Work out the finished part from the listing and answer in its coordinate system (mm). Face numbers are marked on the shaded views. Round coordinates to 2 decimals unless told otherwise and drop trailing zeros. Write each loop counter-clockwise with the first axis right and the second up, starting at its lowest first coordinate (ties: lowest second). Pieces come first, ordered by that corner, then holes. Notation, with made-up numbers: (65, -37.75) -> (84, -37.75) arc R8 cw to (84, -24.75) -> close; hole circle Ø8 at (32.25, 84.5). An arc over 180 degrees is marked (long way). One line per item, written item: value.
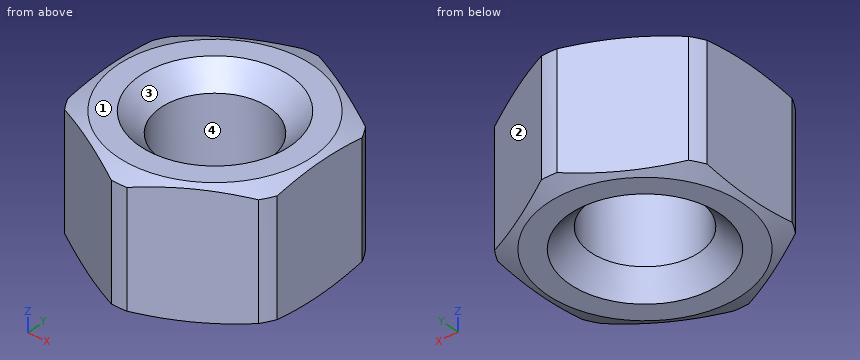
```python
from build123d import *

# Parameters (mm, degrees)
SKETCH_2_OUTSIDE_W  = 36.874
SKETCH_2_OUTSIDE_H  = 36.874
CUT_EXTRUDE_1_DEPTH = 15.8


with BuildPart() as part:
    # Эскиз1 → Повернуть1 (revolve)
    with BuildSketch(Plane(origin=(0, 0, 0), x_dir=(0, 0, -1), z_dir=(1, 0, 0))):
        Polygon((-5.017949192, 6.267949192), (5.017949192, 6.267949192), (7.4, 8.65), (7.4, 11.25), (6.626563252, 13.375), (-6.626563252, 13.375), (-7.4, 11.25), (-7.4, 8.65), align=None)
    revolve(axis=Axis((0, 0, 152.740188543), (0, 0, -1)))

    # Эскиз2 outside → Вырез-Вытянуть1 (cut, through all)
    with BuildSketch(Plane.XY.offset(7.4)):
        Rectangle(SKETCH_2_OUTSIDE_W, SKETCH_2_OUTSIDE_H)
        Polygon((0, -13.856406461), (12, -6.92820323), (12, 6.92820323), (0, 13.856406461), (-12, 6.92820323), (-12, -6.92820323), align=None, mode=Mode.SUBTRACT)
    extrude(amount=-CUT_EXTRUDE_1_DEPTH, mode=Mode.SUBTRACT)


solid = part.part
```
(1) For a pull along Y with two mould halves and no side action, classify the marked faces 1, 2, 3 and 4 as pulls with the +Y half, pulls with the -Y half, needs draft (parallel to the pull), parting line crosses it, or undercut.
Reported:
face 1: needs draft
face 2: pulls with the +Y half
face 3: undercut
face 4: undercut
(2) Consider probe 1 along X at (y, z) = (0, 1); probe 2 along Y at (x, z) = (0.5, 3.5); probe 3 along X at (y, z) = (2, 0.5). Determine where each line is inside the solid, lowest interval first.
Reported:
probe 1: x = -12 to -6.27, 6.27 to 12
probe 2: y = -13.37 to -6.25, 6.25 to 13.37
probe 3: x = -12 to -5.94, 5.94 to 12
(3) Find section A-A on z = 3.25. Give the vertices of the cut face in (x, y) (3 decimals), plus the area to 3 significant figures.
Reported:
outline: (-12, -5.907) arc R13.375 ccw to (-11.115, -7.439) -> (-0.885, -13.346) arc R13.375 ccw to (0.885, -13.346) -> (11.115, -7.439) arc R13.375 ccw to (12, -5.907) -> (12, 5.907) arc R13.375 ccw to (11.115, 7.439) -> (0.885, 13.346) arc R13.375 ccw to (-0.885, 13.346) -> (-11.115, 7.439) arc R13.375 ccw to (-12, 5.907) -> close; hole circle Ø12.536 at (0, 0)
area: 373 mm2
(4) Find section C-C on x = 0. Give the vertices of the cut face in (y, z) (3 decimals), plus the area to 3 significant figures.
Reported:
outline: (-13.375, -6.627) -> (-11.25, -7.4) -> (-8.65, -7.4) -> (-6.268, -5.018) -> (-6.268, 5.018) -> (-8.65, 7.4) -> (-11.25, 7.4) -> (-13.375, 6.627) -> close; (6.268, -5.018) -> (8.65, -7.4) -> (11.25, -7.4) -> (13.375, -6.627) -> (13.375, 6.627) -> (11.25, 7.4) -> (8.65, 7.4) -> (6.268, 5.018) -> close
area: 196 mm2
(5) Flat-ended cylindrical pins translate along their axes: pin 1 Ø2 at (y, z) = (-10, 4.5) entering from +X; pin 2 Ø1 at (x, z) = (8, -6) entering from +Y; pin 3 Ø5 at (x, y) = (4, -3.5) entering from +Z. Find the tip coordinate at first contact, or state that the pin passes through.
Reported:
pin 1: stops at x = 8.41
pin 2: stops at y = 9.53
pin 3: stops at z = 6.57
(6) Find section B-B on y = 0. Give the vertices of the cut face in (x, z), plus the area to 3 significant figures.
Reported:
outline: (-12, -7.13) -> (-11.25, -7.4) -> (-8.65, -7.4) -> (-6.27, -5.02) -> (-6.27, 5.02) -> (-8.65, 7.4) -> (-11.25, 7.4) -> (-12, 7.13) -> close; (6.27, -5.02) -> (8.65, -7.4) -> (11.25, -7.4) -> (12, -7.13) -> (12, 7.13) -> (11.25, 7.4) -> (8.65, 7.4) -> (6.27, 5.02) -> close
area: 158 mm2
